Job drawing, mm, ordinate dimensions from the low corner. One solid piece. Give positions to 0.01 mm unless a question says otherwise; leave off trailing zeros. Order: outer loops, then holes, each group sorted by start corner. A loop starts at its lowest first (then second) coordinate and runs counter-clockwise, first axis right, second up. Notation, with made-up numbers: M 55.5,86.25 L 70.5,86.25 A24 cw 70.5,99.25 Z; hole C -13,4.5 d4. An arc over 180 degrees is marked long. One line per item, written item: value. Start each with the question number.
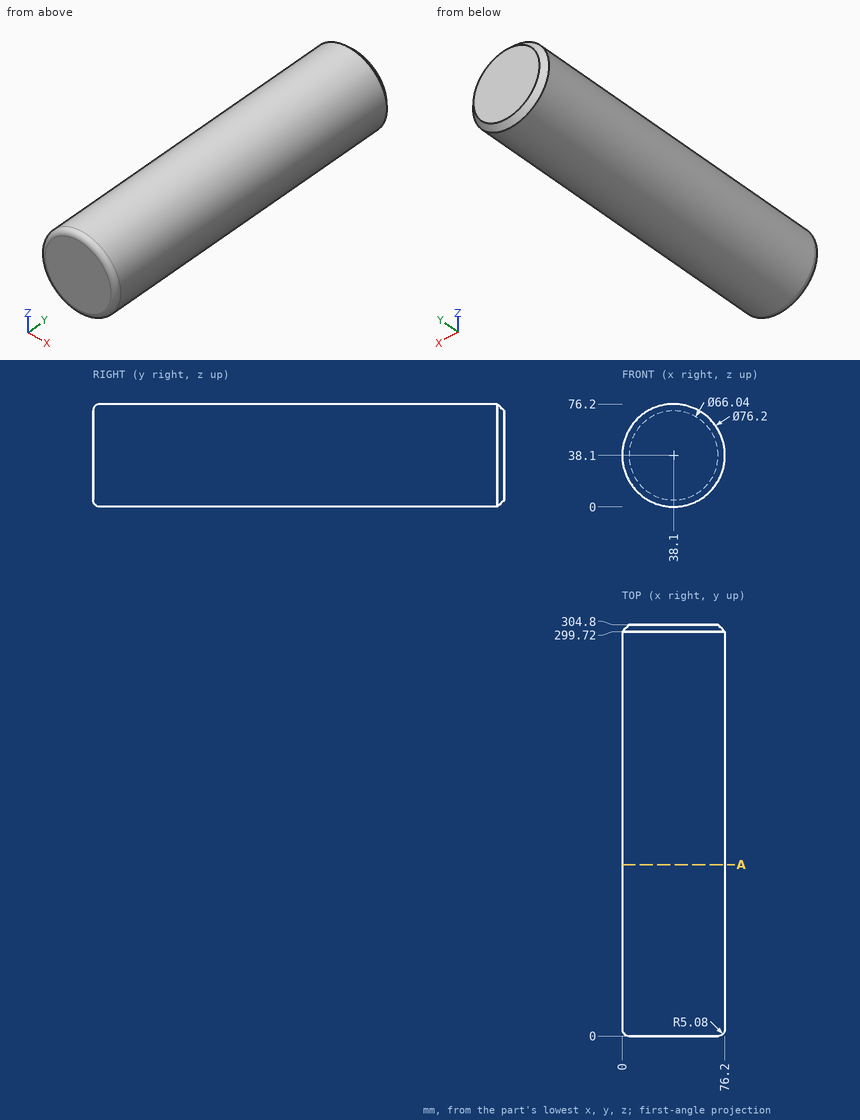
1) Slice it at A-A (y = 127). List the corners of the cut face in (x, z).
2) Drill centre lines: line 1 (X direction, y = 250.5, z = 38.5); line 2 (Z direction, x = 9, y = 199.5); line 3 (Y direction, x = 46.5, z = 72.5). Where is each one in solid material? Low to high.
3) Drop flat-ended pins along their axis: P1, Ø5, axis at x = 12, y = 81.5, coming from the -Z side; P2, Ø8, axis at y = 195, z = 44, coming from the +X side; P3, Ø1.5, axis at y = 238.5, z = 24, coming from the +X side. Give the stop position or say it passes through.
Results list:
1. outline: C 38.1,38.1 d76.2
2. line 1: x = 0 to 76.2
2. line 2: z = 13.51 to 62.69
2. line 3: y = 0.6 to 302.41
3. P1: stops at z = 8.19
3. P2: stops at x = 76.15
3. P3: stops at x = 73.78
